For this review, take the finished solid that the model builds, in its own axes (mm). A direction names the side the tool comes from. Give positions to 0.01 mm unless a question says otherwise; leave off trailing zeros. Order: outer loops, then holes, each group sorted by start corner. A loop starts at its lowest first (then second) coordinate and runs counter-clockwise, first axis right, second up. Notation, with made-up numbers: (9.25, 2) - (65.25, 2) arc R16 cw to (65.25, 12) - close; hole circle Ø4 at (-14, 34). An arc over 180 degrees is marked (long way). Use a Markdown table: item, result. Add a question column.
1) We need section D-D on x = -8.5. Write out the cut boundary in (y, z).
2) We need section C-C on y = -1.5. Write out the cut boundary in (x, z), then the cut area to 3 significant figures.
3) Machinability: for faces 4 (the face through (-40, -1, 15)), 5 (the face through (33.53, 3.34, 15.21)), 6 (the face through (36.904, 6.161, 14.79)), which of the approach directions +Z, -Z, +X, -X, +Y, -Y give a long, thin tool a straight path to every point of the face, cutting with its end or side? Answer none if there is none.
4) We need section A-A on x = 0. Write out the cut boundary in (y, z).
5) We need section B-B on z = 15. Write out the cut boundary in (x, y).
6) Mouldability with a two-part tool opening along X and no side actions: class faces 1 (the face through (-39.503, 4.961, 14.79)), 2 (the face through (40, -1, 15)), 3 (the face through (-1.08, 0.04, 19.88)) as released by +X, released by -X, zero draft, split by the parting line, or undercut.
7) Wall thickness on L1, parallel to X at y = -0.4, z = 15; L2, parallel to X at y = 1.5, z = 11.75; L3, parallel to X at y = 1.5, z = 21.75: over which ranges is each line inside the solid? List them lowest first.
8) Clearance check with flat-ended pins moving along their axes: P1, Ø3, axis at x = 30, y = 4.5, coming from the -Z side; P2, Ø2, axis at y = 1.5, z = 9.5, coming from the -X side; P3, Ø9, axis at x = 10.5, z = 10, coming from the +Y side; P4, Ø3, axis at y = 0, z = 17, coming from the -X side. State where each tip first meets the part, or that it passes through.
```python
from build123d import *

# Parameters (mm, degrees)
BOSS_EXTRUDE1_DEPTH = 30
FILLET1_R           = 5
SKETCH2_R           = 5
CUT_EXTRUDE1_DEPTH  = 10


with BuildPart() as part:
    # Sketch1 → Boss-Extrude1 (new body)
    with BuildSketch(Plane.XY):
        Polygon((40, -2.528830443), (40, 2.528830443), (36.805899489, 2.528830443), (36.02578828, 0.838966186), (35.708014936, 0.9856635), (36.4204046, 2.528830443), (34, 2.528830443), (-34, 2.528830443), (-36.4204046, 2.528830443), (-35.708014936, 0.9856635), (-36.02578828, 0.838966186), (-36.805899489, 2.528830443), (-40, 2.528830443), (-40, -2.528830443), align=None)
        Polygon((-40.838270366, 4.344678122), (-40, 2.528830443), (-36.805899489, 2.528830443), (-38.205291231, 5.560170152), align=None)
        Polygon((-36.4204046, 2.528830443), (-34, 2.528830443), (-35.892316174, 6.627935069), (-37.887517887, 5.706867466), align=None)
        Polygon((34, 2.528830443), (36.4204046, 2.528830443), (37.887517887, 5.706867466), (35.892316174, 6.627935069), align=None)
        Polygon((36.805899489, 2.528830443), (40, 2.528830443), (40.838270366, 4.344678122), (38.205291231, 5.560170152), align=None)
    extrude(amount=BOSS_EXTRUDE1_DEPTH)

    # Fillet1
    fillet1_edges = [part.edges().sort_by_distance(p)[0] for p in [
        (34, 2.528830443, 15),
        (40, 2.528830443, 15),
        (-40, 2.528830443, 15),
        (-34, 2.528830443, 15),
    ]]
    fillet(fillet1_edges, radius=FILLET1_R)

    # Sketch2 → Cut-Extrude1 (cut)
    with BuildSketch(Plane(origin=(0, 2.528830443, 0), x_dir=(1, 0, 0), z_dir=(0, 1, 0))):
        with Locations((0, -15)):
            Circle(SKETCH2_R)
    extrude(amount=-CUT_EXTRUDE1_DEPTH, mode=Mode.SUBTRACT)


solid = part.part
```
Checked values:
| question | item | result |
|---|---|---|
| 1 | outline | (-2.53, 0) - (2.53, 0) - (2.53, 30) - (-2.53, 30) - close |
| 2 | outline | (-40, 0) - (40, 0) - (40, 30) - (-40, 30) - close; hole circle Ø10 at (0, 15) |
| 2 | area | 2,320 mm² |
| 3 | face 4 | +Z, -Z, -X, -Y |
| 3 | face 5 | +Z, -Z, +Y |
| 3 | face 6 | +Z, -Z, +X, +Y |
| 4 | outline | (-2.53, 0) - (2.53, 0) - (2.53, 10) - (-2.53, 10) - close; (-2.53, 20) - (2.53, 20) - (2.53, 30) - (-2.53, 30) - close |
| 5 | outline | (-40.84, 4.34) - (-40.46, 3.53) arc R5 cw to (-40, 1.43) - (-40, -2.53) - (-5, -2.53) - (-5, 2.53) - (-30.8, 2.53) arc R5 cw to (-35.34, 5.43) - (-35.89, 6.63) - (-37.89, 5.71) - (-35.71, 0.99) - (-36.03, 0.84) - (-38.21, 5.56) - close; (5, -2.53) - (40, -2.53) - (40, 1.43) arc R5 cw to (40.46, 3.53) - (40.84, 4.34) - (38.21, 5.56) - (36.03, 0.84) - (35.71, 0.99) - (37.89, 5.71) - (35.89, 6.63) - (35.34, 5.43) arc R5 cw to (30.8, 2.53) - (5, 2.53) - close |
| 6 | face 1 | released by -X |
| 6 | face 2 | released by +X |
| 6 | face 3 | undercut |
| 7 | L1 | -40 to -5, 5 to 40 |
| 7 | L2 | -40 to -36.33, -35.95 to -3.8, 3.8 to 35.95, 36.33 to 40 |
| 7 | L3 | -40 to -36.33, -35.95 to 35.95, 36.33 to 40 |
| 8 | P1 | through |
| 8 | P2 | x = -40.12 |
| 8 | P3 | y = 2.53 |
| 8 | P4 | x = -40 |
